```python
from build123d import *

# Parameters (mm, degrees)
CUT_EXTRUDE1_DEPTH      = 30
CUT_EXTRUDE1_DEPTH_BACK = 5
BOSS_EXTRUDE1_DEPTH     = 73
CUT_EXTRUDE2_DEPTH      = 20
CUT_EXTRUDE2_DEPTH_BACK = 20
SKETCH5_W               = 66.529199046
SKETCH5_H               = 33.448723993
BOSS_EXTRUDE3_DEPTH     = 20
CUT_EXTRUDE3_DEPTH      = 20
CIRPATTERN1_COUNT       = 6


with BuildPart() as part:
    # Sketch1 → Revolve1 (revolve)
    with BuildSketch(Plane.XY, mode=Mode.PRIVATE) as revolve1_sk:
        Polygon((9.842999887, 11.113), (29.842999887, 11.113), (39.842999887, 18), (66.842999887, 18), (66.842999887, 22), (39.842999887, 22), (29.842999887, 15.113), (9.842999887, 15.113), align=None)
    revolve(revolve1_sk.sketch.rotate(Axis((-3.645367966, 0, 0), (1, 0, 0)), 90), axis=Axis((-3.645367966, 0, 0), (1, 0, 0)))

    # Sketch2 → Cut-Extrude1 (cut, two sides: drawn at the far end of the back side and taken through both)
    with BuildSketch(Plane(origin=(46.7775, 0, 0), x_dir=(0, 0, -1), z_dir=(1, 0, 0)).offset(-CUT_EXTRUDE1_DEPTH_BACK)):
        with BuildLine():
            Line((-5, 8.659676688), (-14.270871629, 14.012216918))
            ThreePointArc((-14.270871629, 14.012216918), (-15.866085859, 12.176506869), (-17.226698597, 10.160750732))
            Line((-17.226698597, 10.160750732), (-17.412817554, 9.838383242))
            ThreePointArc((-17.412817554, 9.838383242), (-18.478009625, 7.652657074), (-19.270095188, 5.353824003))
            Line((-19.270095188, 5.353824003), (-9.999, 0.001154701))
            Line((-9.999, 0.001154701), (-5, 2.887328696))
            Line((-5, 2.887328696), (-5, 8.659676688))
        make_face()
        with BuildLine():
            Line((0.001, 5.774657392), (5, 8.660831388))
            Line((5, 8.660831388), (5, 19.364916731))
            ThreePointArc((5, 19.364916731), (0.001032782, 19.999999973), (-4.998, 19.365433019))
            Line((-4.998, 19.365433019), (-4.998, 8.660831388))
            Line((-4.998, 8.660831388), (0.001, 5.774657392))
        make_face()
        with BuildLine():
            Line((10.001, 0.001154701), (19.270371629, 5.352828906))
            ThreePointArc((19.270371629, 5.352828906), (17.320766265, 9.999552789), (14.271595188, 14.011479965))
            Line((14.271595188, 14.011479965), (5.002, 8.659676688))
            Line((5.002, 8.659676688), (5.002, 2.887328696))
            Line((5.002, 2.887328696), (10.001, 0.001154701))
        make_face()
        with BuildLine():
            Line((19.270371629, -5.352828906), (10.001, -0.001154701))
            Line((10.001, -0.001154701), (5.002, -2.887328696))
            Line((5.002, -2.887328696), (5.002, -8.659676688))
            Line((5.002, -8.659676688), (14.271595188, -14.011479965))
            ThreePointArc((14.271595188, -14.011479965), (17.320766265, -9.999552789), (19.270371629, -5.352828906))
        make_face()
        with BuildLine():
            Line((5, -8.660831388), (0.001, -5.774657392))
            Line((0.001, -5.774657392), (-4.998, -8.660831388))
            Line((-4.998, -8.660831388), (-4.998, -19.365433019))
            ThreePointArc((-4.998, -19.365433019), (0.001032782, -19.999999973), (5, -19.364916731))
            Line((5, -19.364916731), (5, -8.660831388))
        make_face()
        with BuildLine():
            Line((-14.270871629, -14.012216918), (-5, -8.659676688))
            Line((-5, -8.659676688), (-5, -2.887328696))
            Line((-5, -2.887328696), (-9.999, -0.001154701))
            Line((-9.999, -0.001154701), (-19.270095188, -5.353824003))
            ThreePointArc((-19.270095188, -5.353824003), (-18.478009625, -7.652657074), (-17.412817554, -9.838383242))
            Line((-17.412817554, -9.838383242), (-17.226698597, -10.160750732))
            ThreePointArc((-17.226698597, -10.160750732), (-15.866085859, -12.176506869), (-14.270871629, -14.012216918))
        make_face()
    extrude(amount=CUT_EXTRUDE1_DEPTH + CUT_EXTRUDE1_DEPTH_BACK, mode=Mode.SUBTRACT)

    # Sketch3 → Boss-Extrude1 (add)
    with BuildSketch(Plane(origin=(-43.2225, 0, 0), x_dir=(0, 0, -1), z_dir=(1, 0, 0))):
        with BuildLine():
            Line((10.03247637, 2.905284302), (10.603848258, 3.325232492))
            ThreePointArc((10.603848258, 3.325232492), (9.677413399, 5.58840998), (8.18031613, 7.522047395))
            Line((8.18031613, 7.522047395), (7.531056114, 7.236900729))
            ThreePointArc((7.531056114, 7.236900729), (8.562885859, 4.944693552), (10.03247637, 2.905284302))
        make_face()
        with BuildLine():
            Line((7.532288195, -7.235737248), (8.18165994, -7.520585723))
            ThreePointArc((8.18165994, -7.520585723), (9.678411709, -5.586680857), (10.604442198, -3.323337882))
            Line((10.604442198, -3.323337882), (10.032867932, -2.903635548))
            ThreePointArc((10.032867932, -2.903635548), (8.56367316, -4.943329907), (7.532288195, -7.235737248))
        make_face()
        with BuildLine():
            Line((-2.500188174, -10.14102155), (-2.422188317, -10.845818215))
            ThreePointArc((-2.422188317, -10.845818215), (0.00099831, -11.175090837), (2.424126068, -10.845385277))
            Line((2.424126068, -10.845385277), (2.501811819, -10.140536276))
            ThreePointArc((2.501811819, -10.140536276), (0.000787301, -9.88802346), (-2.500188174, -10.14102155))
        make_face()
        with BuildLine():
            Line((-10.03247637, -2.905284302), (-10.603848258, -3.325232492))
            ThreePointArc((-10.603848258, -3.325232492), (-9.677413399, -5.58840998), (-8.18031613, -7.522047395))
            Line((-8.18031613, -7.522047395), (-7.531056114, -7.236900729))
            ThreePointArc((-7.531056114, -7.236900729), (-8.562885859, -4.944693552), (-10.03247637, -2.905284302))
        make_face()
        with BuildLine():
            Line((-7.532288195, 7.235737248), (-8.18165994, 7.520585723))
            ThreePointArc((-8.18165994, 7.520585723), (-9.678411709, 5.586680857), (-10.604442198, 3.323337882))
            Line((-10.604442198, 3.323337882), (-10.032867932, 2.903635548))
            ThreePointArc((-10.032867932, 2.903635548), (-8.56367316, 4.943329907), (-7.532288195, 7.235737248))
        make_face()
        with BuildLine():
            Line((2.500188174, 10.14102155), (2.422188317, 10.845818215))
            ThreePointArc((2.422188317, 10.845818215), (-0.00099831, 11.175090837), (-2.424126068, 10.845385277))
            Line((-2.424126068, 10.845385277), (-2.501811819, 10.140536276))
            ThreePointArc((-2.501811819, 10.140536276), (-0.000787301, 9.88802346), (2.500188174, 10.14102155))
        make_face()
    extrude(amount=BOSS_EXTRUDE1_DEPTH)

    # Sketch5 → Cut-Extrude2 (cut, two sides: drawn at the far end of the back side and taken through both)
    with BuildSketch(Plane.XY.offset(-CUT_EXTRUDE2_DEPTH_BACK)):
        with Locations((-23.421599636, -1.611361997)):
            Rectangle(SKETCH5_W, SKETCH5_H)
    extrude(amount=CUT_EXTRUDE2_DEPTH + CUT_EXTRUDE2_DEPTH_BACK, mode=Mode.SUBTRACT)

    # Sketch6 → Boss-Extrude3 (add)
    with BuildSketch(Plane(origin=(9.7775, 0, 0), x_dir=(0, 0, -1), z_dir=(1, 0, 0))):
        with BuildLine():
            ThreePointArc((2.661916341, 10.789484251), (2.542208375, 10.818315284), (2.422188317, 10.845818215))
            Line((2.422188317, 10.845818215), (2.501811819, 10.140536276))
            Line((2.501811819, 10.140536276), (2.661916341, 10.789484251))
        make_face()
        with BuildLine():
            Line((-2.661916341, 10.789484251), (-2.501811819, 10.140536276))
            Line((-2.501811819, 10.140536276), (-2.424126068, 10.845385277))
            ThreePointArc((-2.424126068, 10.845385277), (-2.543174803, 10.818088136), (-2.661916341, 10.789484251))
        make_face()
    extrude(amount=BOSS_EXTRUDE3_DEPTH)

    # Sketch7 → Cut-Extrude3 (cut, symmetric)
    with BuildSketch(Plane(origin=(9.842999887, 0, 0), x_dir=(0, 0, -1), z_dir=(1, 0, 0))):
        with BuildLine():
            Line((2.422188317, 10.845818215), (2.422188317, 10.1253438))
            Line((2.422188317, 10.1253438), (2.532529127, 10.096901244))
            Line((2.532529127, 10.096901244), (2.554732852, 10.240216199))
            Line((2.554732852, 10.240216199), (3.06458678, 10.682091409))
            ThreePointArc((3.06458678, 10.682091409), (2.74460869, 10.76874608), (2.422188317, 10.845818215))
        make_face()
        with BuildLine():
            Line((-2.532529127, 10.096901244), (-2.422188317, 10.1253438))
            Line((-2.422188317, 10.1253438), (-2.422188317, 10.845818215))
            ThreePointArc((-2.422188317, 10.845818215), (-2.74460869, 10.76874608), (-3.06458678, 10.682091409))
            Line((-3.06458678, 10.682091409), (-2.554732852, 10.240216199))
            Line((-2.554732852, 10.240216199), (-2.532529127, 10.096901244))
        make_face()
    cut_extrude3 = extrude(amount=CUT_EXTRUDE3_DEPTH, both=True, mode=Mode.SUBTRACT)

    # CirPattern1: Cut-Extrude3 ×6 about axis
    cirpattern1_axis = Axis((0, 0, 0), (1, 0, 0))
    for i in range(1, CIRPATTERN1_COUNT):
        add(cut_extrude3.rotate(cirpattern1_axis, i * 360 / CIRPATTERN1_COUNT), mode=Mode.SUBTRACT)


solid = part.part
```
Read the model definition and answer for the solid it produces. Units are mm, in the model's axes. A direction names the side the tool comes from. Give positions to 0.01 mm unless a question says otherwise; leave off trailing zeros. Loops run counter-clockwise (first coordinate to the right, second up) from the corner with the lowest first, then second, coordinate; pieces in that order, holes last.
Item 1: Each of these flat-tipped pins is pushed along its axis until it touches: pin 1 Ø1 at (x, y) = (55.5, 18) entering from -Z; pin 2 Ø1.5 at (y, z) = (6, -10) entering from +X; pin 3 Ø2.5 at (x, y) = (53.5, -18.5) entering from +Z; pin 4 Ø1.5 at (y, z) = (-16, -16.5) entering from -X. Where does it stop, or does it pass through?
Item 2: The part is cut by section B-B (z = 0). Write down the section's boundary in (x, y), and give its area (3 significant figures).
Item 3: For faces 3 (the cylindrical face through (19.671, 4.914, 8.581)), 4 (the cylindrical face through (54.135, 9.938, -17.356)), determine the directions among +Z, -Z, +X, -X, +Y, -Y from which every point of the face is accessible in a straight line to the end or side of a thin tool.
Item 4: The part is cut by section A-A (y = 0). Write down the section's boundary in (x, z), and give its area (3 significant figures).
Item 5: Find the intervals of material crossed by line 1 along Y through (x, z) = (20.5, 0); line 2 along Y through (x, z) = (53.75, 0); line 3 along Z through (x, y) = (39.5, 5.5), in increasing order.
Item 6: The mould has two halves that part along Z. Classify faces 1 (the flat face through (9.843, -4, 10)), 2 (the flat face through (54.135, 13.5, -13.386)): released by +Z, released by -Z, zero draft, split by the parting line, or undercut.
Taken from the geometry:
1. pin 1: stops at z = -13.33
1. pin 2: stops at x = 31.73
1. pin 3: stops at z = 13.65
1. pin 4: passes through
2. outline: (9.84, -15.11) - (29.84, -15.11) - (39.84, -22) - (66.84, -22) - (66.84, -20) - (41.78, -20) - (41.78, -18) - (39.84, -18) - (29.84, -11.11) - (29.78, -11.11) - (29.78, -9.89) - (9.84, -9.89) - close; (9.84, 9.89) - (29.78, 9.89) - (29.78, 11.11) - (29.84, 11.11) - (39.84, 18) - (41.78, 18) - (41.78, 20) - (66.84, 20) - (66.84, 22) - (39.84, 22) - (29.84, 15.11) - (9.84, 15.11) - close
2. area: 405 mm2
3. face 3: +X, -X
3. face 4: +X
4. outline: (9.84, -15.11) - (29.84, -15.11) - (39.84, -22) - (66.84, -22) - (66.84, -18) - (39.84, -18) - (29.84, -11.11) - (9.84, -11.11) - close; (9.84, 11.11) - (29.84, 11.11) - (39.84, 18) - (66.84, 18) - (66.84, 22) - (39.84, 22) - (29.84, 15.11) - (9.84, 15.11) - close
4. area: 456 mm2
5. line 1: y = -15.11 to -9.89, 9.89 to 15.11
5. line 2: y = -22 to -20, 20 to 22
5. line 3: z = -21.06 to -16.89, 16.89 to 21.06
6. face 1: zero draft
6. face 2: undercut
